For this review, take the finished solid that the model builds, in its own axes (mm). A direction names the side the tool comes from. Coordinates: 2 decimals unless noted, no trailing zeros. Loops run counter-clockwise (first coordinate to the right, second up) from the corner with the lowest first, then second, coordinate; pieces in that order, holes last. Notation, with made-up numbers: (88.25, 6) -> (100.25, 6) arc R7 cw to (100.25, 10) -> close; hole circle Ø6 at (49, 47.25). An arc over 180 degrees is marked (long way). Use a Markdown table: item, result.
from build123d import *

# Parameters (mm, degrees)
BASE_FLANGE1_DEPTH     = 6
SKETCHED_START         = -25
SKETCHED_BEND1_DEPTH   = 50
SKETCHED_BEND1_2_DEPTH = 50
SKETCH8_R              = 3
CUT_EXTRUDE1_DEPTH     = 81.54392997
FILLET1_R              = 10
SKETCH10_R             = 3
CUT_EXTRUDE2_DEPTH     = 88.139684731


# Read off the part's stored shape, not the designer's step: Sketched Bend1
# Sheet-metal steps are written as plain solids
with BuildPart() as part:
    # Sketch1 → Base-Flange1 (new body)
    with BuildSketch(Plane(origin=(0, 0, 0), x_dir=(1, 0, 0), z_dir=(0, 1, 0))):
        Polygon((25, 20), (67.5, 20), (67.5, -20), (-67.5, -20), (-67.5, 20), (-25, 20), (-25, 58), (25, 58), align=None)
    extrude(amount=-BASE_FLANGE1_DEPTH)

    # Sketched Bend1 outline → Sketched Bend1 (cut)
    with BuildSketch(Plane.YZ.offset(SKETCHED_START)):
        with BuildLine():
            Line((0, -58), (0, -30.677078252))
            ThreePointArc((0, -30.677078252), (-4.397247359, -26.123724357), (-6, -20))
            Line((-6, -20), (-6, -58))
            Line((-6, -58), (0, -58))
        make_face()
    extrude(amount=SKETCHED_BEND1_DEPTH, mode=Mode.SUBTRACT)

    # Sketched Bend1 2 outline → Sketched Bend1 2 (add)
    with BuildSketch(Plane.YZ.offset(SKETCHED_START)):
        with BuildLine():
            Line((6.5, -32.5), (29.577434895, -32.5))
            Line((29.577434895, -32.5), (29.577434895, -26.5))
            Line((29.577434895, -26.5), (6.5, -26.5))
            ThreePointArc((6.5, -26.5), (1.903805922, -24.596194078), (0, -20))
            Line((0, -20), (0, -30.677078252))
            ThreePointArc((0, -30.677078252), (3.124609515, -32.035644523), (6.5, -32.5))
        make_face()
    extrude(amount=SKETCHED_BEND1_2_DEPTH)

    # Sketch8 → Cut-Extrude1 (cut, through all)
    with BuildSketch(Plane(origin=(0, 0, 0), x_dir=(1, 0, 0), z_dir=(0, 1, 0))):
        with Locations(Location((-55, -7.5, 0), (0, 0, 270))):
            Circle(SKETCH8_R)
        with Locations(Location((55, -7.5, 0), (0, 0, 90))):
            Circle(SKETCH8_R)
    extrude(amount=-CUT_EXTRUDE1_DEPTH, mode=Mode.SUBTRACT)

    # Fillet1
    fillet1_edges = [part.edges().sort_by_distance(p)[0] for p in [
        (-67.5, -3, 20),
        (67.5, -3, 20),
        (67.5, -3, -20),
        (-67.5, -3, -20),
    ]]
    fillet(fillet1_edges, radius=FILLET1_R)

    # Sketch10 → Cut-Extrude2 (cut, through all)
    with BuildSketch(Plane.XY.offset(-26.5)):
        with Locations((-7.5, 19.577434895)):
            Circle(SKETCH10_R)
        with Locations(Location((7.5, 19.577434895, 0), (0, 0, 180))):
            Circle(SKETCH10_R)
    extrude(amount=-CUT_EXTRUDE2_DEPTH, mode=Mode.SUBTRACT)


solid = part.part
(1) Mouldability with a two-part tool opening along Z and no side actions: class faces 6 (the face through (-52.47, -2.96, 9.11)), 7 (the face through (1, -3, 20)), 8 (the face through (0, 18, -32.5)), 9 (the face through (6.12, 22.24, -29.46)) as pulls with the +Z half, pulls with the -Z half, needs draft (parallel to the pull), parting line crosses it, or undercut.
Found:
| item | result |
|---|---|
| face 6 | undercut |
| face 7 | pulls with the +Z half |
| face 8 | pulls with the -Z half |
| face 9 | needs draft |
(2) Take a section at B-B on x = -23. Write out the cut boundary in (y, z), plus the area to 3 significant figures.
Found:
| item | result |
|---|---|
| outline | (-6, -20) arc R12.5 ccw to (6.5, -32.5) -> (29.58, -32.5) -> (29.58, -26.5) -> (6.5, -26.5) arc R6.5 cw to (0, -20) -> (0, 20) -> (-6, 20) -> close |
| area | 468 mm^2 |
(3) For line 1 along X through (y, z) = (-4, 7.5); line 2 along Y through (x, z) = (-21, -15); line 3 along X through (y, z) = (-1, -26.5), list the stretches that pass through material, from the lowest coordinate up.
Found:
| item | result |
|---|---|
| line 1 | x = -67.5 to -58, -52 to 52, 58 to 67.5 |
| line 2 | y = -6 to 0 |
| line 3 | x = -25 to 25 |
(4) Take a section at D-D on z = -3.5. Write out the cut boundary in (x, y), plus the area to 3 significant figures.
Found:
| item | result |
|---|---|
| outline | (-67.5, -6) -> (67.5, -6) -> (67.5, 0) -> (-67.5, 0) -> close |
| area | 810 mm^2 |
(5) For pin 1 Ø20 at (x, z) = (27.5, 10) entering from +Y; pin 2 Ø5 at (x, y) = (46, -4) entering from -Z; pin 3 Ø7 at (x, z) = (55, 7.5) entering from -Y; pin 4 Ø11.5 at (x, y) = (7, 20) entering from +Z, all flat-tipped, find the tip position at first contact; note any pin that passes through.
Found:
| item | result |
|---|---|
| pin 1 | stops at y = 0 |
| pin 2 | stops at z = -20 |
| pin 3 | stops at y = -6 |
| pin 4 | stops at z = -26.5 |
(6) Take a section at A-A on x = -7.5. Write out the cut boundary in (y, z), plus the area to 3 significant figures.
Found:
| item | result |
|---|---|
| outline | (-6, -20) arc R12.5 ccw to (6.5, -32.5) -> (16.58, -32.5) -> (16.58, -26.5) -> (6.5, -26.5) arc R6.5 cw to (0, -20) -> (0, 20) -> (-6, 20) -> close; (22.58, -32.5) -> (29.58, -32.5) -> (29.58, -26.5) -> (22.58, -26.5) -> close |
| area | 432 mm^2 |
(7) Take a section at C-C on x = 55. Write out the cut boundary in (y, z).
Found:
| item | result |
|---|---|
| outline | (-6, -20) -> (0, -20) -> (0, 4.5) -> (-6, 4.5) -> close; (-6, 10.5) -> (0, 10.5) -> (0, 20) -> (-6, 20) -> close |
(8) For faces 1 (the face through (67.5, -3, 0)), 2 (the face through (41, -3, -20)), 3 (the face through (-25, 12, -28)), 4 (the face through (0, 18, -26.5)), 5 (the face through (1, -6, 0)), list the 3-axis set-ups (+Z, -Z, +X, -X, +Y, -Y) from which the entire face can be reached by the end or side of a thin tool; tool diameter is ignored.
Found:
| item | result |
|---|---|
| face 1 | +Z, -Z, +X, +Y, -Y |
| face 2 | -Z, +X, +Y, -Y |
| face 3 | -Z, -X, +Y, -Y |
| face 4 | +Z, +X, -X, +Y |
| face 5 | +Z, -Z, +X, -X, -Y |
